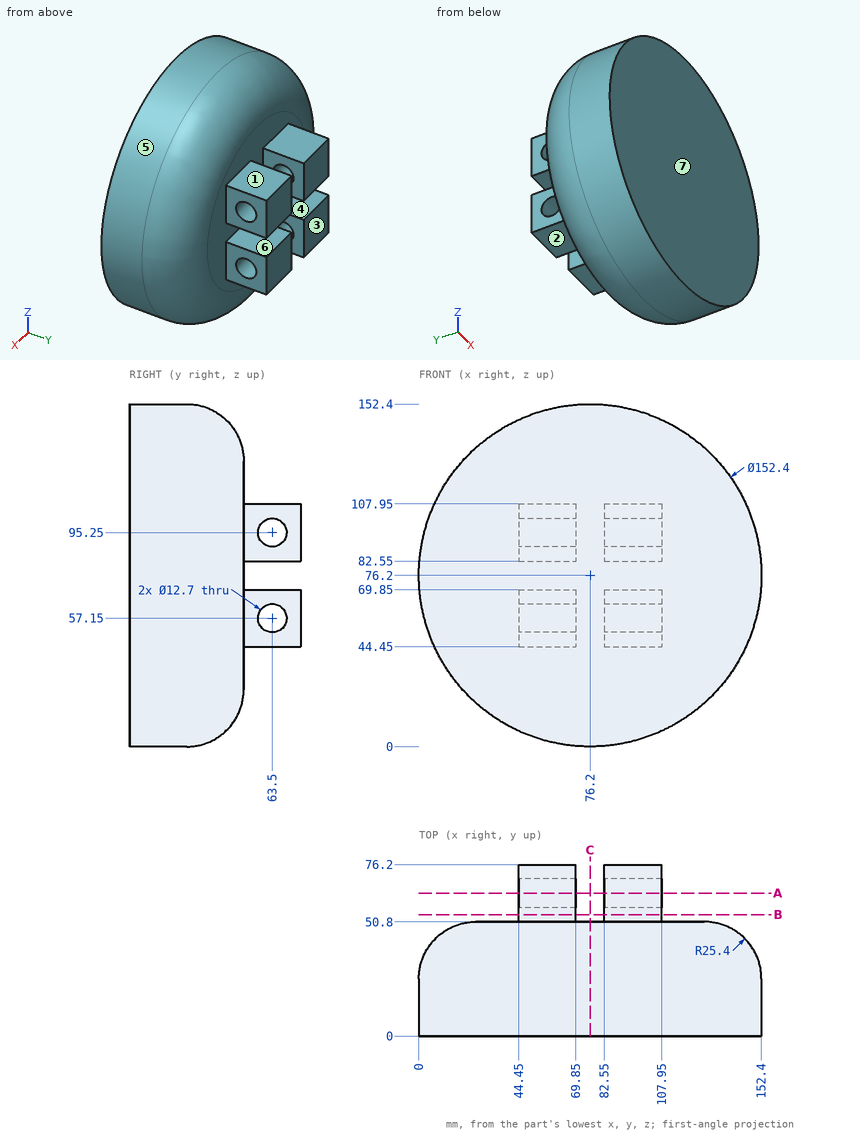
Drawing for the job (mm, zero at the part's lowest x, y, z). A direction names the side the tool comes from. Coordinates: 2 decimals unless noted, no trailing zeros. Write each loop counter-clockwise with the first axis right and the second up, starting at its lowest first coordinate (ties: lowest second). Pieces come first, ordered by that corner, then holes. Notation, with made-up numbers: (81.5, 69) - (119.5, 69) arc R21 ccw to (119.5, 75) - close; hole circle Ø3 at (72, 56). An arc over 180 degrees is marked (long way). Write each question's results on one line, items separated by ' | '. Start each with the question number.
1) Cut at B-B (y = 54). Write the cut outline in (x, z).
2) Cut at C-C (x = 76.2). Write the cut outline in (y, z).
3) 3-axis set-ups, long thin cutter, end or side, ignore diameter. For the marked faces 1, 2 and 3: which of +Z, -Z, +X, -X, +Y, -Y reach the whole face in a straight line?
4) Flat gauge pins, fed straight in: P1, Ø16.5, axis at y = 63.5, z = 57.15, coming from the -X side; P2, Ø12.5, axis at y = 58.5, z = 53.5, coming from the +X side; P3, Ø12.5, axis at x = 97.5, y = 58.5, coming from the -Z side; P4, Ø7.5, axis at y = 62, z = 93.5, coming from the +X side. Where does each tip first touch, or does it go through?
5) Cut at A-A (y = 63.5). Count the separate pieces of the cut face and the enclosed holes in it, then the cut area to 3 significant figures.
6) Probe line 1 along Z through (x, y) = (51, 63); line 2 along Y through (x, z) = (60.75, 95.25); line 3 along Z through (x, y) = (104, 67). List the from-to ranges inside material, lowest first. Write a range as from..to.
7) Mould opens along Z. For the marked faces 4, 5, 6 and 7 say: pulls with the +Z half, pulls with the -Z half, needs draft (parallel to the pull), parting line crosses it, or undercut.
Returned:
1) outline: (44.45, 44.45) - (69.85, 44.45) - (69.85, 69.85) - (44.45, 69.85) - close; (44.45, 82.55) - (69.85, 82.55) - (69.85, 107.95) - (44.45, 107.95) - close; (82.55, 44.45) - (107.95, 44.45) - (107.95, 69.85) - (82.55, 69.85) - close; (82.55, 82.55) - (107.95, 82.55) - (107.95, 107.95) - (82.55, 107.95) - close
2) outline: (0, 0) - (25.4, 0) arc R25.4 ccw to (50.8, 25.4) - (50.8, 127) arc R25.4 ccw to (25.4, 152.4) - (0, 152.4) - close
3) face 1: +Z, +X, -X, +Y | face 2: -Z, +X, -X, +Y | face 3: +Z, -Z, +X, -X, +Y
4) P1: x = 44.45 | P2: x = 107.95 | P3: z = 44.45 | P4: through
5) separate pieces: 8 | enclosed holes: 0 | area: 1,290 mm^2
6) line 1: 44.45..50.82, 63.48..69.85, 82.55..88.92, 101.58..107.95 | line 2: 0..57.15, 69.85..76.2 | line 3: 44.45..51.85, 62.45..69.85, 82.55..89.95, 100.55..107.95
7) face 4: undercut | face 5: parting line crosses it | face 6: undercut | face 7: needs draft
